The model under review builds one solid part; all positions refer to its coordinate system, in mm. Face numbers are marked on the shaded views. Coordinates: 2 decimals unless noted, no trailing zeros. Loops run counter-clockwise (first coordinate to the right, second up) from the corner with the lowest first, then second, coordinate; pieces in that order, holes last. Notation, with made-up numbers: M -25,-2 L 30,-2 A21 cw 30,13 Z; hole C 89.5,-7 d6. An arc over 180 degrees is marked long. Return JSON: item names as keys, results as strings.
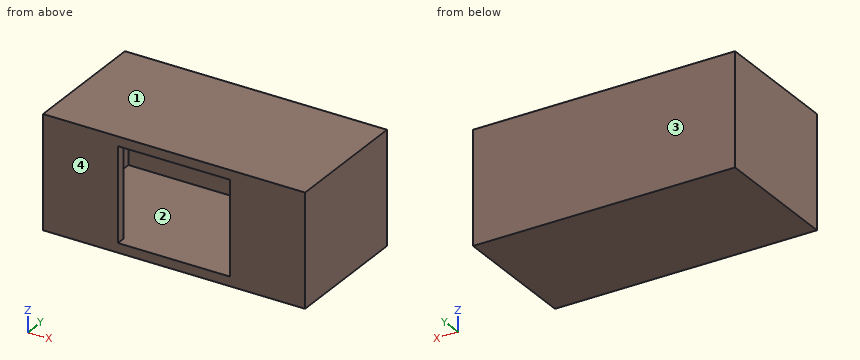
```python
from build123d import *

# Parameters (mm, degrees)
IZIM1_W                     = 140
IZIM1_H                     = 70
Y_KSEKLIK_EKSTR_ZYON1_DEPTH = 60
IZIM10_W                    = 130
IZIM10_H                    = 50
KES_EKSTR_ZYON6_DEPTH       = 65
IZIM12_W                    = 35
IZIM12_H                    = 50
Y_KSEKLIK_EKSTR_ZYON3_DEPTH = 5


with BuildPart() as part:
    # Çizim1 → Yükseklik-Ekstrüzyon1 (new body)
    with BuildSketch(Plane.XY):
        with Locations((70, 35)):
            Rectangle(IZIM1_W, IZIM1_H)
    extrude(amount=Y_KSEKLIK_EKSTR_ZYON1_DEPTH)

    # Çizim10 → Kes-Ekstrüzyon6 (cut)
    with BuildSketch(Plane.XZ):
        with Locations((70, 30)):
            Rectangle(IZIM10_W, IZIM10_H)
    extrude(amount=-KES_EKSTR_ZYON6_DEPTH, mode=Mode.SUBTRACT)

    # Çizim12 → Yükseklik-Ekstrüzyon3 (add)
    with BuildSketch(Plane.XZ):
        with Locations((22.5, 30)):
            Rectangle(IZIM12_W, IZIM12_H)
        with Locations((117.5, 30)):
            Rectangle(IZIM12_W, IZIM12_H)
    extrude(amount=-Y_KSEKLIK_EKSTR_ZYON3_DEPTH)


solid = part.part
```
1. Add section A-A on x = 21. Give the boundary of the cut face in (y, z), plus the area to 3 significant figures.
Check values:
{"outline": "M 0,0 L 70,0 L 70,60 L 0,60 Z; hole M 5,5 L 65,5 L 65,55 L 5,55 Z", "area": "1,200 mm²"}
2. Add section D-D on x = 66.5. Give the boundary of the cut face in (y, z).
Check values:
{"outline": "M 0,0 L 70,0 L 70,60 L 0,60 L 0,55 L 65,55 L 65,5 L 0,5 Z"}
3. Add section C-C on z = 38.5. Give the boundary of the cut face in (x, y), plus the area to 3 significant figures.
Check values:
{"outline": "M 0,0 L 40,0 L 40,5 L 5,5 L 5,65 L 135,65 L 135,5 L 100,5 L 100,0 L 140,0 L 140,70 L 0,70 Z", "area": "1,700 mm²"}
4. Insertion check: pin 1 Ø2 at (x, z) = (70, 39) entering from -Y. The pin has a flat end and moves straight along its axis. Give the tip position at first contact, or say it passes through.
Check values:
{"pin 1": "y = 65"}
5. Add section B-B on y = 43. Give the boundary of the cut face in (x, z).
Check values:
{"outline": "M 0,0 L 140,0 L 140,60 L 0,60 Z; hole M 5,5 L 135,5 L 135,55 L 5,55 Z"}
6. To check wall thickness, follow line 1 (Z direction, x = 127, y = 55); line 2 (Y direction, x = 18.5, z = 29.5); line 3 (X direction, y = 9.5, z = 48.5). State the ranges of each line that lie inside material, in increasing order.
Check values:
{"line 1": "0 to 5, 55 to 60", "line 2": "0 to 5, 65 to 70", "line 3": "0 to 5, 135 to 140"}
7. The part is to be moulded in two halves that separate along Y. For the marked faces 1, 2, 3 and 4, say which applies: released by +Y, released by -Y, zero draft, split by the parting line, or undercut.
Check values:
{"face 1": "zero draft", "face 2": "undercut", "face 3": "released by +Y", "face 4": "released by -Y"}
